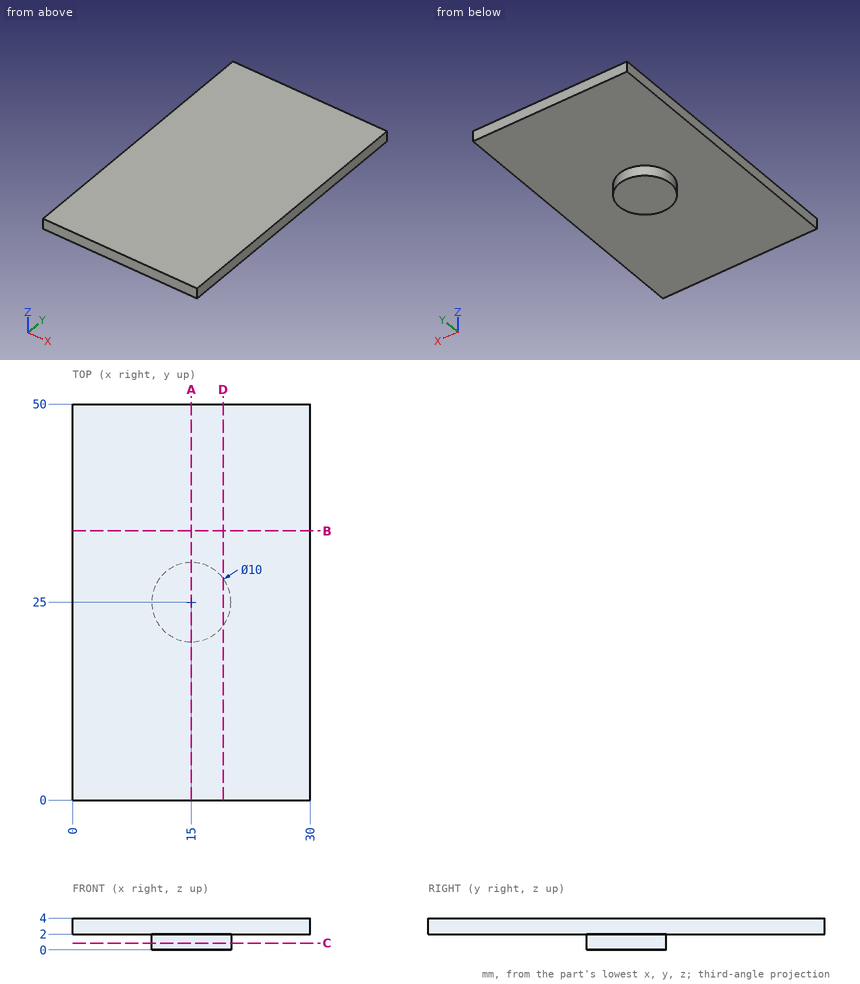
Geometry check sheet. Reference: drawing and pictorial views, mm from the part's lowest x, y, z. Give positions to 0.01 mm unless a question says otherwise; leave off trailing zeros. Write each loop counter-clockwise with the first axis right and the second up, starting at its lowest first coordinate (ties: lowest second). Pieces come first, ordered by that corner, then holes. Notation, with made-up numbers: (72, 49.25) -> (108, 49.25) arc R30 cw to (108, 76.25) -> close; hole circle Ø8 at (21.25, 59.5). An arc over 180 degrees is marked (long way). One line per question, with ' | ' between items.
Item 1: Sectioned sample at B-B, the plane y = 34. Record the boundary of the cut face in (x, z).
Determined:
outline: (0, 2) -> (30, 2) -> (30, 4) -> (0, 4) -> close
Item 2: Depth check by flat-ended pin: pin 1 (9 mm diameter, centred on x = 18.5, y = 36, fed in from -Z). Enter the tip coordinate at first touch or a pass-through.
Determined:
pin 1: z = 2
Item 3: Sectioned sample at A-A, the plane x = 15. Record the boundary of the cut face in (y, z), plus the area to 3 significant figures.
Determined:
outline: (0, 2) -> (20, 2) -> (20, 0) -> (30, 0) -> (30, 2) -> (50, 2) -> (50, 4) -> (0, 4) -> close | area: 120 mm^2
Item 4: Sectioned sample at C-C, the plane z = 0.85. Record the boundary of the cut face in (x, y).
Determined:
outline: circle Ø10 at (15, 25)
Item 5: Scan lines: line 1 along Z through (x, y) = (2, 40); line 2 along Y through (x, z) = (15, 1); line 3 along X through (y, z) = (26.5, 0.5). Record each from-to range of solid material in increasing order.
Determined:
line 1: 2 to 4 | line 2: 20 to 30 | line 3: 10.23 to 19.77
Item 6: Sectioned sample at D-D, the plane x = 19. Record the boundary of the cut face in (y, z), plus the area to 3 significant figures.
Determined:
outline: (0, 2) -> (22, 2) -> (22, 0) -> (28, 0) -> (28, 2) -> (50, 2) -> (50, 4) -> (0, 4) -> close | area: 112 mm^2
